Here's the drawing with two shaded views (mm, measured from the low corner). I have some questions. A direction names the side the tool comes from. Coordinates: 2 decimals unless noted, no trailing zeros. Loops run counter-clockwise (first coordinate to the right, second up) from the corner with the lowest first, then second, coordinate; pieces in that order, holes last. Notation, with made-up numbers: (84, 60) -> (140, 60) arc R27 cw to (140, 98) -> close; hole circle Ø6 at (-31, 19.5). An arc over 180 degrees is marked (long way). Answer as a JSON object with one key per item and string values. Group by question number.
1) I want a section at C-C (z = 20.5). Write out the boundary of the cut face in (x, y), then the cut area to 3 significant figures.
2) I'm going to push flat-ended pins straight in: pin 1 (8 mm diameter, centred on y = 27.5, z = 11.5, fed in from -X); pin 2 (12 mm diameter, centred on y = 37.5, z = 33, fed in from -X); pin 3 (8 mm diameter, centred on y = 15.5, z = 47.5, fed in from -X). Where does each tip first touch, or does it pass through?
3) I want a section at D-D (y = 33). Write out the boundary of the cut face in (x, z) (1 decimal), then the cut area to 3 significant figures.
4) I need wall thicknesses on probe 1 along Z at (x, y) = (51, 8.89) (1 decimal); probe 2 along Y at (x, z) = (3, 70); probe 3 along X at (y, z) = (42.5, 33). Which ranges of each line are inside material? Lowest first, please. Write a range as [from, to].
5) I want a section at B-B (x = 22). Write out the boundary of the cut face in (y, z).
6) Which directions (+Z, -Z, +X, -X, +Y, -Y) give clear straight access to the entire face, cutting with the end or side of a thin tool? Please do the marked faces 1 and 2.
7) If we mould it in two halves opening along Z, with no side actions, what happens to the marked faces 3, 4 and 5? For each: +Z half, -Z half, draft (parallel to the pull), parting line (faces both ways), or undercut.
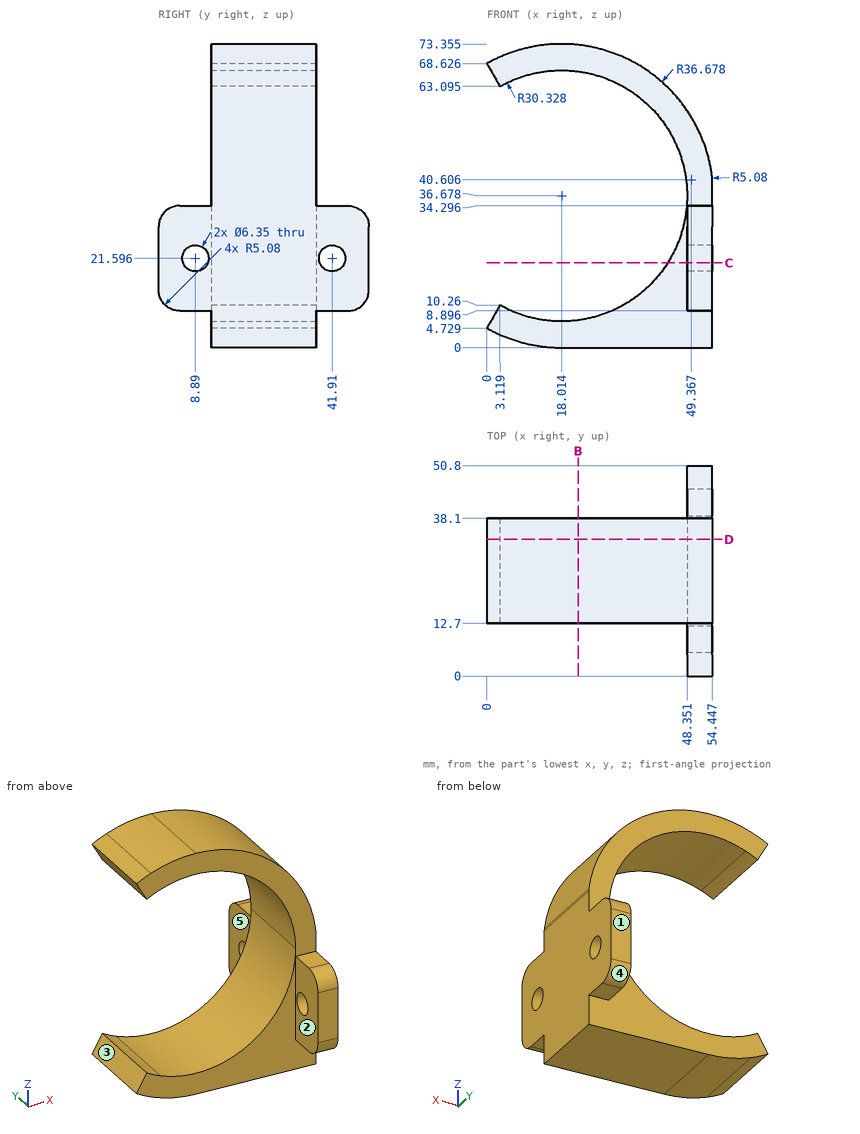
Determined:
{
 "1": {"outline": "(43.67, 12.7) -> (48.35, 12.7) -> (48.35, 11.87) -> (54.45, 11.87) -> (54.45, 38.93) -> (48.35, 38.93) -> (48.35, 38.1) -> (43.67, 38.1) -> close; (48.35, 0) -> (54.45, 0) -> (54.45, 5.91) -> (48.35, 5.91) -> close; (48.35, 44.89) -> (54.45, 44.89) -> (54.45, 50.8) -> (48.35, 50.8) -> close", "area": "356 mm^2"},
 "2": {"pin 1": "x = 1.56", "pin 2": "x = 46.76", "pin 3": "x = 44.47"},
 "3": {"outline": "(0, 4.7) arc R36.7 ccw to (18, 0) -> (54.4, 0) -> (54.4, 40.6) arc R5.1 ccw to (54.4, 41.2) arc R36.7 ccw to (0, 68.6) -> (3.1, 63.1) arc R30.3 cw (long way) to (3.1, 10.3) -> close", "area": "1,170 mm^2"},
 "4": {"probe 1": "[8.9, 18.4], [24.8, 34.3]", "probe 2": "[12.7, 38.1]", "probe 3": "[48.35, 54.45]"},
 "5": {"outline": "(12.7, 0) -> (38.1, 0) -> (38.1, 6.61) -> (12.7, 6.61) -> close; (12.7, 66.74) -> (38.1, 66.74) -> (38.1, 73.14) -> (12.7, 73.14) -> close"},
 "6": {"face 1": "+Z, -Z, +X, -X, +Y", "face 2": "+Z, -Z, -X, -Y"},
 "7": {"face 3": "undercut", "face 4": "-Z half", "face 5": "draft"}
}
